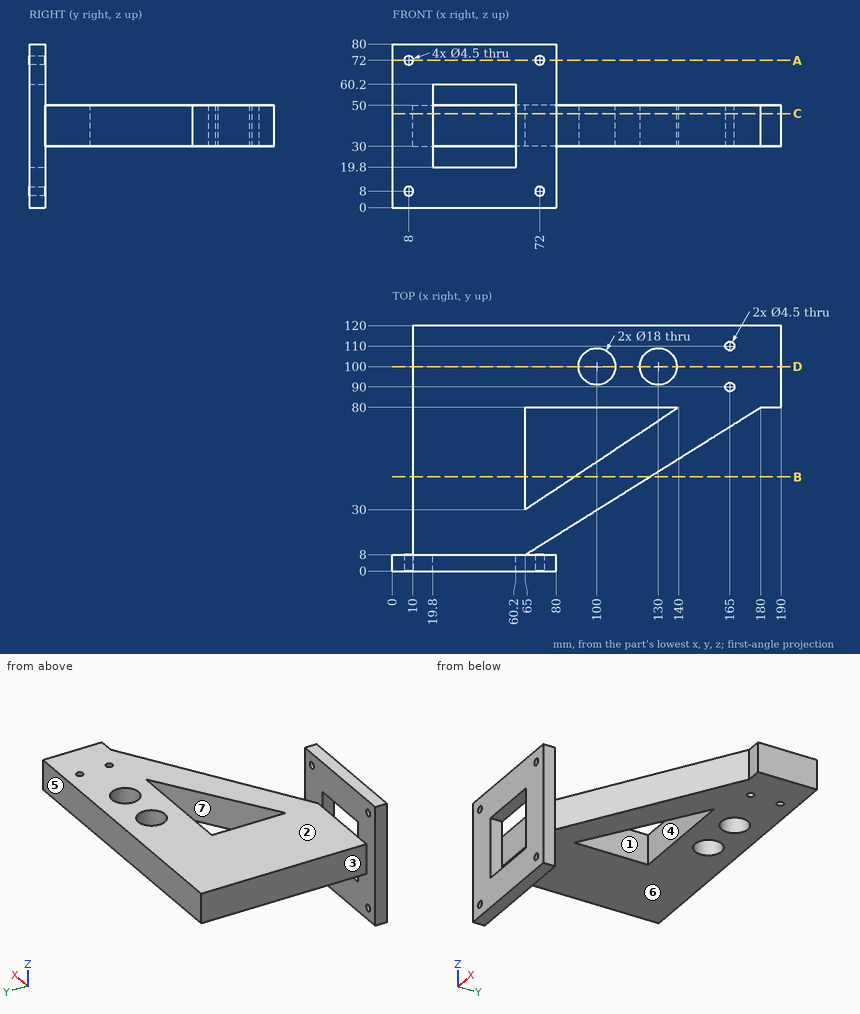
Here's the drawing with two shaded views (mm, measured from the low corner). I have some questions. A direction names the side the tool comes from. Give positions to 0.01 mm unless a question says otherwise; leave off trailing zeros. Loops run counter-clockwise (first coordinate to the right, second up) from the corner with the lowest first, then second, coordinate; pieces in that order, holes last. Notation, with made-up numbers: M 63,37.25 L 80,37.25 A15 ccw 80,48.25 Z; hole C 6,-33.5 d7. An arc over 180 degrees is marked long. Use one line per item in the form item = value. Start each with the question number.
Q1. Which directions (+Z, -Z, +X, -X, +Y, -Y) give clear straight access to the entire face, cutting with the end or side of a thin tool? Please do the marked faces 1, 2 and 3.
Q2. Will these pins go through, and if not, where does the flat tip stop? pin 1 Ø6 at (y, z) = (46, 38.5) entering from +X; pin 2 Ø20.5 at (x, y) = (130, 100) entering from +Z; pin 3 Ø6 at (x, y) = (21.5, 97.5) entering from -Z.
Q3. If we section it at B-B (y = 46): Write out the boundary of the cut face in (x, z).
Q4. Thinking about a two-plate mould opening in Y: for the marked faces 4, 5, 6 and 7, which applies, +Y half, -Y half, draft (parallel to the pull), parting line (faces both ways), or undercut?
Q5. If we section it at A-A (z = 72): Write out the boundary of the cut face in (x, y), then the cut area to 3 significant figures.
Q6. If we section it at C-C (z = 46): Write out the boundary of the cut face in (x, y).
Q7. I need wall thicknesses on line 1 along X through (y, z) = (2.5, 8); line 2 along X through (y, z) = (100, 35). Which ranges of each line are inside material? Lowest first, please.
Q8. If we section it at D-D (y = 100): Write out the boundary of the cut face in (x, z).
Taken from the geometry:
q1.face_1 = +Z, -Z
q1.face_2 = +Z, +X, -X, +Y
q1.face_3 = +Z, -Z, -X, +Y
q2.pin_1 = 130.49
q2.pin_2 = 50
q2.pin_3 = 30
q3.outline = M 10,30 L 65,30 L 65,50 L 10,50 Z; M 89,30 L 125.69,30 L 125.69,50 L 89,50 Z
q4.face_4 = undercut
q4.face_5 = +Y half
q4.face_6 = draft
q4.face_7 = undercut
q5.outline = M 0,0 L 5.75,0 L 5.75,8 L 0,8 Z; M 10.25,0 L 69.75,0 L 69.75,8 L 10.25,8 Z; M 74.25,0 L 80,0 L 80,8 L 74.25,8 Z
q5.area = 568 mm^2
q6.outline = M 0,0 L 19.8,0 L 19.8,8 L 60.2,8 L 60.2,0 L 80,0 L 80,8 L 65,8 L 180,80 L 190,80 L 190,120 L 10,120 L 10,8 L 0,8 Z; hole M 65,30 L 140,80 L 65,80 Z; hole C 100,100 d18; hole C 130,100 d18; hole C 165,90 d4.5; hole C 165,110 d4.5
q7.line_1 = 0 to 5.75, 10.25 to 69.75, 74.25 to 80
q7.line_2 = 10 to 91, 109 to 121, 139 to 190
q8.outline = M 10,30 L 91,30 L 91,50 L 10,50 Z; M 109,30 L 121,30 L 121,50 L 109,50 Z; M 139,30 L 190,30 L 190,50 L 139,50 Z
